Build history of the part. All positions in model axes, mm. Round coordinates to 2 decimals unless told otherwise and drop trailing zeros. Write each loop counter-clockwise with the first axis right and the second up, starting at its lowest first coordinate (ties: lowest second). Pieces come first, ordered by that corner, then holes. Notation, with made-up numbers: (28, 23) -> (63, 23) arc R17 ccw to (63, 34) -> close; hole circle Ø1 at (-27.75, 47.25). An arc over 180 degrees is marked (long way). Answer in a Markdown table with one row per item. Add a question column.
from build123d import *

# Parameters (mm, degrees)
F0_R     = 9
F1_DEPTH = 3
F3_D     = 1.778
F3_DEPTH = 15
F3_TIP   = 0.5341650903


# Not quite as in the source:
# - a feature names something its author has since deleted; it is built from what else it names


with BuildPart() as f1:
    # F0 (on Front) → F1 (new body)
    with BuildSketch(Plane.XZ):
        Circle(F0_R)
    extrude(amount=F1_DEPTH)

    # F3
    with Locations(Plane.XZ.offset(3)):
        with Locations((-3.5267115138, 4.8541019662), (-5.7063390978, 1.8541019662), (-5.7063390978, -1.8541019662), (-3.5267115138, -4.8541019662), (0, -6), (3.5267115138, -4.8541019662), (5.7063390978, -1.8541019662), (0, 6), (-2.0225424859, 1.4694631307), (-2.0225424859, -1.4694631307), (0.7725424859, -2.3776412907), (2.5, 0), (0.7725424859, 2.3776412907), (3.5267115138, 4.8541019662), (5.7063390978, 1.8541019662)):
            Hole(F3_D / 2, depth=F3_DEPTH)
            with Locations((0, 0, -(F3_DEPTH + F3_TIP / 2))):  # 118° drill point
                Cone(0, F3_D / 2, F3_TIP, mode=Mode.SUBTRACT)


solid = f1.part
(1) Probe line 1 along Z through (x, y) = (-4, -0.3); line 2 along X through (y, z) = (-1.5, 1.25); line 3 along Z through (x, y) = (-0.25, -2.8). List the from-to ranges inside material, lowest first.
(2) Saw through at A-A (z = -6). List the corners of the cut face in (x, y), plus the area to 3 significant figures.
(3) Mould opens along Z. For faces 1 (the face through (0.36, -1.48, 1.59)), 2 (the face through (-1.172, -1.479, 8.923)), 3 (the face through (0, 0, 0)) say: pulls with the +Z half, pulls with the -Z half, needs draft (parallel to the pull), parting line crosses it, or undercut.
(4) Drop flat-ended pins along their axis: P1, Ø1.1, axis at x = -3.53, z = -4.85, coming from the +Y side; P2, Ø1, axis at x = -4, y = -2.5, coming from the -Z side. Give the stop position or say it passes through.
(5) Saw through at B-B (y = -1.65). Count the separate pieces of the cut face and the enclosed holes in it, plus the area to 3 significant figures.
(6) Saw through at C-C (z = 3.5). List the corners of the cut face in (x, y), plus the area to 3 significant figures.
Answer sheet:
| question | item | result |
|---|---|---|
| 1 | line 1 | z = -8.06 to -5.61, -4.1 to 4.1, 5.61 to 8.06 |
| 1 | line 2 | x = -8.91 to -6.36, -5.05 to -2.88, -1.16 to 5.05, 6.36 to 8.91 |
| 1 | line 3 | z = -9 to -6.85, -5.15 to 5.15, 6.85 to 9 |
| 2 | outline | (-6.71, -3) -> (-0.89, -3) -> (-0.89, 0) -> (-6.71, 0) -> close; (0.89, -3) -> (6.71, -3) -> (6.71, 0) -> (0.89, 0) -> close |
| 2 | area | 34.9 mm² |
| 3 | face 1 | undercut |
| 3 | face 2 | parting line crosses it |
| 3 | face 3 | needs draft |
| 4 | P1 | passes through |
| 4 | P2 | stops at z = -8.29 |
| 5 | separate pieces | 1 |
| 5 | enclosed holes | 15 |
| 5 | area | 217 mm² |
| 6 | outline | (-8.29, -3) -> (8.29, -3) -> (8.29, 0) -> (-8.29, 0) -> close |
| 6 | area | 49.7 mm² |
